Work out the finished part from the listing and answer in its coordinate system (mm). A direction names the side the tool comes from. Coordinates: 2 decimals unless noted, no trailing zeros. Write each loop counter-clockwise with the first axis right and the second up, starting at its lowest first coordinate (ties: lowest second). Pieces come first, ordered by that corner, then holes. Notation, with made-up numbers: (41.25, 76.5) - (66.25, 76.5) arc R25 ccw to (66.25, 98.5) - close; hole circle Ø3 at (44, 4). An arc over 180 degrees is marked (long way). Use a Markdown table: item, result. Add a question column.
(1) For a pull along X with two mould halves and no side action, classify faces 1 (the face through (11.5, -9.6, -2.1)), 2 (the face through (5, -5, 0)), 3 (the face through (5.3, -0.5, -1)), 4 (the face through (-2, -5, -2)) as released by +X, released by -X, zero draft, split by the parting line, or undercut.
(2) A tool of negligible diameter and unlimited length cuts with its end or side. For faces 5 (the face through (10.5, -5, -2)), 6 (the face through (5, 0, 0)), from which of +Z, -Z, +X, -X, +Y, -Y can it reach the whole face along a straight path? Write none if from no direction.
(3) The part is cut by section B-B, the plane x = 6. Give the vertices of the cut face in (y, z), then the cut area to 3 significant figures.
(4) The part is cut by section C-C, the plane y = -5.5. Give the vertices of the cut face in (x, z), then the cut area to 3 significant figures.
(5) Given pin 1 Ø0.5 at (x, y) = (5.5, -0.5) entering from -Z; pin 2 Ø1.5 at (x, y) = (5, -4.5) entering from -Z; pin 3 Ø1.5 at (x, z) = (6, -1.5) entering from -Y; pin 4 Ø2 at (x, z) = (10, -0.5) entering from -Y, each flat-ended and moving along its own axis, determine where each tip first touches the part or whether it passes through.
(6) The part is cut by section A-A, the plane z = -1.7. Give the vertices of the cut face in (x, y).
(7) Find the intervals of material crossed by line 1 (X direction, y = -2.75, z = -3.85); line 2 (Z direction, x = 2.25, y = -4.25); line 3 (Y direction, x = 0.25, z = -0.8), in increasing order. Write a range as from..to.
from build123d import *

# Parameters (mm, degrees)
SKETCH_1_W      = 10.5
SKETCH_1_H      = 8.6
EXTRUDE_1_DEPTH = 0.6
SKETCH_2_W      = 2
SKETCH_2_H      = 8.6
EXTRUDE_2_DEPTH = 5.4
EXTRUDE_3_DEPTH = 1
SKETCH_4_W      = 10.5
SKETCH_4_H      = 1
EXTRUDE_4_DEPTH = 1
CHAMFER_1_SIZE  = 0.4


with BuildPart() as part:
    # Эскиз1 → Бобышка-Вытянуть1 (new body)
    with BuildSketch(Plane.XY):
        with Locations((5.25, -4.3)):
            Rectangle(SKETCH_1_W, SKETCH_1_H)
    extrude(amount=EXTRUDE_1_DEPTH)

    # Эскиз2 → Бобышка-Вытянуть2 (add)
    with BuildSketch(Plane.XY.offset(0.6)):
        with Locations((-1, -4.3)):
            Rectangle(SKETCH_2_W, SKETCH_2_H)
        with Locations((11.5, -4.3)):
            Rectangle(SKETCH_2_W, SKETCH_2_H)
    extrude(amount=-EXTRUDE_2_DEPTH)

    # Эскиз3 → Бобышка-Вытянуть3 (add)
    with BuildSketch(Plane.XZ.offset(8.6)):
        Polygon((10.5, 0), (10.5, -4.8), (12.5, -4.8), (12.5, 0.6), (-2, 0.6), (-2, -4.8), (0, -4.8), (0, 0), align=None)
    extrude(amount=EXTRUDE_3_DEPTH)

    # Эскиз4 → Бобышка-Вытянуть4 (add)
    with BuildSketch(Plane(origin=(0, 0, 0), x_dir=(-1, 0, 0), z_dir=(0, 0, -1))):
        with Locations((-5.25, -0.5)):
            Rectangle(SKETCH_4_W, SKETCH_4_H)
    extrude(amount=EXTRUDE_4_DEPTH)

    # Фаска1
    # the kernel refuses this chamfer: 0.4 mm, written as the material it takes off along each edge
    with BuildSketch(Plane(origin=(0, -9.6, -5.828673195), x_dir=(0.02749587661058617, 0.9996219169112966, 0), z_dir=(0, 0, 1)), Plane(origin=(10.5, -9.6, 0), x_dir=(-0.027495876610587302, 0.9996219169112966, 0), z_dir=(0, 0, -1))) as chamfer_1_piece_1:
        Polygon((CHAMFER_1_SIZE * 0.999621916911, CHAMFER_1_SIZE * 0.0274958766106), (-CHAMFER_1_SIZE * 0.0274958766106, CHAMFER_1_SIZE * 0.999621916911), (0, 0), align=None)
    extrude(amount=5.828673195, mode=Mode.SUBTRACT)
    with BuildSketch(Plane(origin=(0, -9.6, 0), x_dir=(0, 0.9996219169112968, -0.027495876610582035), z_dir=(1, 0, 0))) as chamfer_1_piece_2:
        Polygon((CHAMFER_1_SIZE * 0.999621916911, CHAMFER_1_SIZE * 0.0274958766106), (-CHAMFER_1_SIZE * 0.0274958766106, CHAMFER_1_SIZE * 0.999621916911), (0, 0), align=None)
    extrude(amount=10.5, mode=Mode.SUBTRACT)
    with BuildSketch(Plane(origin=(9.471326805, -9.6, -4.8), x_dir=(0, 0.9996219169112966, -0.027495876610587302), z_dir=(1, 0, 0)), Plane(origin=(-3.028673195, -9.6, -4.8), x_dir=(0, 0.9996219169112966, -0.027495876610587302), z_dir=(1, 0, 0))) as chamfer_1_piece_3:
        Polygon((CHAMFER_1_SIZE * 0.999621916911, CHAMFER_1_SIZE * 0.0274958766106), (-CHAMFER_1_SIZE * 0.0274958766106, CHAMFER_1_SIZE * 0.999621916911), (0, 0), align=None)
    extrude(amount=4.05734639, mode=Mode.SUBTRACT)
    with BuildSketch(Plane(origin=(12.5, -9.6, -5.828673195), x_dir=(0.027495876610587302, 0.9996219169112966, 0), z_dir=(0, 0, 1)), Plane(origin=(-2, -9.6, 1.628673195), x_dir=(-0.027495876610586223, 0.9996219169112966, 0), z_dir=(0, 0, -1))) as chamfer_1_piece_4:
        Polygon((CHAMFER_1_SIZE * 0.999621916911, CHAMFER_1_SIZE * 0.0274958766106), (-CHAMFER_1_SIZE * 0.0274958766106, CHAMFER_1_SIZE * 0.999621916911), (0, 0), align=None)
    extrude(amount=7.45734639, mode=Mode.SUBTRACT)
    with BuildSketch(Plane(origin=(13.528673195, -9.6, 0.6), x_dir=(0, 0.9996219169112968, 0.027495876610586226), z_dir=(-1, 0, 0))) as chamfer_1_piece_5:
        Polygon((CHAMFER_1_SIZE * 0.999621916911, CHAMFER_1_SIZE * 0.0274958766106), (-CHAMFER_1_SIZE * 0.0274958766106, CHAMFER_1_SIZE * 0.999621916911), (0, 0), align=None)
    extrude(amount=16.55734639, mode=Mode.SUBTRACT)
    with BuildSketch(Plane(origin=(0, -9.6, -5.828673195), x_dir=(0.02749587661058617, 0.9996219169112966, 0), z_dir=(0, 0, 1))) as chamfer_1_piece_6a_section:
        Polygon((CHAMFER_1_SIZE * 0.999621916911, CHAMFER_1_SIZE * 0.0274958766106), (-CHAMFER_1_SIZE * 0.0274958766106, CHAMFER_1_SIZE * 0.999621916911), (0, 0), align=None)
    chamfer_1_piece_6a = extrude(amount=6.85734639, mode=Mode.PRIVATE)
    chamfer_1_piece_6a = split(chamfer_1_piece_6a, bisect_by=Plane(origin=(-0.131917451, -9.468082549, 0), z_dir=(0, 0, 1)), keep=Keep.TOP, mode=Mode.PRIVATE)
    with BuildSketch(Plane(origin=(-1.028673195, -9.6, 0), x_dir=(0, 0.9996219169112968, -0.027495876610586317), z_dir=(1, 0, 0))) as chamfer_1_piece_6b_section:
        Polygon((CHAMFER_1_SIZE * 0.999621916911, CHAMFER_1_SIZE * 0.0274958766106), (-CHAMFER_1_SIZE * 0.0274958766106, CHAMFER_1_SIZE * 0.999621916911), (0, 0), align=None)
    chamfer_1_piece_6b = extrude(amount=11.528673195, mode=Mode.PRIVATE)
    chamfer_1_piece_6b = split(chamfer_1_piece_6b, bisect_by=Plane(origin=(0, -9.468082549, 0.131917451), z_dir=(-1, 0, 0)), keep=Keep.TOP, mode=Mode.PRIVATE)
    chamfer_1_piece_6 = chamfer_1_piece_6a & chamfer_1_piece_6b
    add(chamfer_1_piece_6, mode=Mode.SUBTRACT)
    with BuildSketch(Plane(origin=(10.5, -9.6, 1.028673195), x_dir=(-0.027495876610587302, 0.9996219169112966, 0), z_dir=(0, 0, -1))) as chamfer_1_piece_7a_section:
        Polygon((CHAMFER_1_SIZE * 0.999621916911, CHAMFER_1_SIZE * 0.0274958766106), (-CHAMFER_1_SIZE * 0.0274958766106, CHAMFER_1_SIZE * 0.999621916911), (0, 0), align=None)
    chamfer_1_piece_7a = extrude(amount=6.85734639, mode=Mode.PRIVATE)
    chamfer_1_piece_7a = split(chamfer_1_piece_7a, bisect_by=Plane(origin=(10.631917451, -9.468082549, 0), z_dir=(0, 0, 1)), keep=Keep.TOP, mode=Mode.PRIVATE)
    with BuildSketch(Plane(origin=(0, -9.6, 0), x_dir=(0, 0.9996219169112968, -0.027495876610582035), z_dir=(1, 0, 0))) as chamfer_1_piece_7b_section:
        Polygon((CHAMFER_1_SIZE * 0.999621916911, CHAMFER_1_SIZE * 0.0274958766106), (-CHAMFER_1_SIZE * 0.0274958766106, CHAMFER_1_SIZE * 0.999621916911), (0, 0), align=None)
    chamfer_1_piece_7b = extrude(amount=11.528673195, mode=Mode.PRIVATE)
    chamfer_1_piece_7b = split(chamfer_1_piece_7b, bisect_by=Plane(origin=(10.5, -9.468082549, 0.131917451), z_dir=(1, 0, 0)), keep=Keep.TOP, mode=Mode.PRIVATE)
    chamfer_1_piece_7 = chamfer_1_piece_7a & chamfer_1_piece_7b
    add(chamfer_1_piece_7, mode=Mode.SUBTRACT)


solid = part.part
Model answer:
| question | item | result |
|---|---|---|
| 1 | face 1 | zero draft |
| 1 | face 2 | undercut |
| 1 | face 3 | undercut |
| 1 | face 4 | released by -X |
| 2 | face 5 | -Z, -Y |
| 2 | face 6 | +Z, -Z, +X, -X, +Y |
| 3 | outline | (-9.5, 0.3) - (-9.2, 0) - (-1, 0) - (-1, -1) - (0, -1) - (0, 0.6) - (-9.2, 0.6) - close |
| 3 | area | 6.61 mm^2 |
| 4 | outline | (-2, -4.8) - (0, -4.8) - (0, 0) - (10.5, 0) - (10.5, -4.8) - (12.5, -4.8) - (12.5, 0.6) - (-2, 0.6) - close |
| 4 | area | 27.9 mm^2 |
| 5 | pin 1 | z = -1 |
| 5 | pin 2 | z = 0 |
| 5 | pin 3 | y = -1 |
| 5 | pin 4 | y = -9.6 |
| 6 | outline | (-2, -9.2) - (-1.6, -9.6) - (-0.4, -9.6) - (0, -9.2) - (0, 0) - (-2, 0) - close; (10.5, -9.2) - (10.9, -9.6) - (12.1, -9.6) - (12.5, -9.2) - (12.5, 0) - (10.5, 0) - close |
| 7 | line 1 | -2..0, 10.5..12.5 |
| 7 | line 2 | 0..0.6 |
| 7 | line 3 | -1..0 |
